from build123d import *

# Parameters (mm, degrees)
SKETCH1_W                     = 99.25
SKETCH1_H                     = 16
BOSS_EXTRUDE1_DEPTH           = 3
SKETCH2_R                     = 2.475
BOSS_EXTRUDE2_DEPTH           = 4.9
BOSS_EXTRUDE2_DRAFT           = 3
BOSS_EXTRUDE2_PROFILE_2_DEPTH = 4.9
BOSS_EXTRUDE2_PROFILE_2_DRAFT = 3


with BuildPart() as part:
    # Sketch1 → Boss-Extrude1 (new body)
    with BuildSketch(Plane(origin=(0, 0, 0), x_dir=(1, 0, 0), z_dir=(0, 1, 0))):
        with Locations((45.45161309, 5.10225193)):
            Rectangle(SKETCH1_W, SKETCH1_H)
    extrude(amount=BOSS_EXTRUDE1_DEPTH)


with BuildPart() as boss_extrude2_tool:
    # Sketch2 → Boss-Extrude2 (with draft: the straight prism first)
    with BuildSketch(Plane(origin=(0, 3, 0), x_dir=(1, 0, 0), z_dir=(0, 1, 0))):
        with Locations((0.82661309, 5.10225193)):
            Circle(SKETCH2_R)
    extrude(amount=BOSS_EXTRUDE2_DEPTH)
    # Boss-Extrude2: the draft: its side faces are tilted about the plane it starts from
    boss_extrude2_sides = [boss_extrude2_tool.faces().sort_by_distance(p)[0] for p in [
        (-1.64838691, 5.45, -5.10225193),
    ]]
    draft(boss_extrude2_sides, Plane(origin=(0, 3, 0), x_dir=(1, 0, 0), z_dir=(0, 1, 0)), BOSS_EXTRUDE2_DRAFT)


with BuildPart() as part_1:
    add(part.part)

    # Boss-Extrude2: add boss_extrude2_tool
    add(boss_extrude2_tool.part)


with BuildPart() as boss_extrude2_profile_2_tool:
    # Sketch2 → Boss-Extrude2 profile 2 (with draft: the straight prism first)
    with BuildSketch(Plane(origin=(0, 3, 0), x_dir=(1, 0, 0), z_dir=(0, 1, 0))):
        with Locations((90.07661309, 5.10225193)):
            Circle(SKETCH2_R)
    extrude(amount=BOSS_EXTRUDE2_PROFILE_2_DEPTH)
    # Boss-Extrude2 profile 2: the draft: its side faces are tilted about the plane it starts from
    boss_extrude2_profile_2_sides = [boss_extrude2_profile_2_tool.faces().sort_by_distance(p)[0] for p in [
        (87.60161309, 5.45, -5.10225193),
    ]]
    draft(boss_extrude2_profile_2_sides, Plane(origin=(0, 3, 0), x_dir=(1, 0, 0), z_dir=(0, 1, 0)), BOSS_EXTRUDE2_PROFILE_2_DRAFT)


with BuildPart() as part_2:
    add(part_1.part)

    # Boss-Extrude2 profile 2: add boss_extrude2_profile_2_tool
    add(boss_extrude2_profile_2_tool.part)


solid = part_2.part
The listing builds one solid part. Answer for the finished solid, in the listing's coordinates (mm). Coordinates: 2 decimals unless noted, no trailing zeros. Loops run counter-clockwise (first coordinate to the right, second up) from the corner with the lowest first, then second, coordinate; pieces in that order, holes last. Notation, with made-up numbers: (-22, 88) -> (29, 88) arc R30 ccw to (29, 119) -> close; hole circle Ø8 at (-33, 23.5). An arc over 180 degrees is marked (long way). Answer in a Markdown table with one row per item. Add a question column.
1. The part is cut by section A-A, the plane y = 4.75. Write down the section's boundary in (x, z), then the cut area to 3 significant figures.
2. The part is cut by section C-C, the plane x = 61. Write down the section's boundary in (y, z), then the cut area to 3 significant figures.
3. A flat-ended cylindrical pin translates along its axis: P1, Ø8, axis at x = 41.5, z = -7, coming from the +Y side. Find the tip coordinate at first contact, or state that the pin passes through.
4. The part is cut by section B-B, the plane z = -9.5. Write down the section's boundary in (x, y), then the cut area to 3 significant figures.
5. Consider line 1 (Y direction, x = 47.5, z = -0.25); line 2 (X direction, y = 4.25, z = -6.5); line 3 (X direction, y = 7.5, z = -3.5). Determine where each line is inside the solid, lowest interval first. Write a range as [from, to].
6. Determine the mould class of faces 1 (the conical face through (3.067, 5.416, -5.808)), 2 (the flat face through (45, 0, -5)), 3 (the flat face through (95.077, 1, -5)) for opening direction X: +X half, -X half, draft (parallel to the pull), parting line (faces both ways), or undercut.
Answer below:
| question | item | result |
|---|---|---|
| 1 | outline | circle Ø4.77 at (0.83, -5.1); circle Ø4.77 at (90.08, -5.1) |
| 1 | area | 35.7 mm2 |
| 2 | outline | (0, -13.1) -> (3, -13.1) -> (3, 2.9) -> (0, 2.9) -> close |
| 2 | area | 48.0 mm2 |
| 3 | P1 | y = 3 |
| 4 | outline | (-4.17, 0) -> (95.08, 0) -> (95.08, 3) -> (-4.17, 3) -> close |
| 4 | area | 298 mm2 |
| 5 | line 1 | [0, 3] |
| 5 | line 2 | [-1.14, 2.79], [88.11, 92.04] |
| 5 | line 3 | [-0.74, 2.39], [88.51, 91.64] |
| 6 | face 1 | undercut |
| 6 | face 2 | draft |
| 6 | face 3 | +X half |
